from build123d import *

# Parameters (mm, degrees)
F1_DEPTH = 400
F2_R     = 15
F3_R     = 15


with BuildPart() as f1:
    # F0 (on Top) → F1 (new body)
    with BuildSketch(Plane.XY):
        Polygon((0, 400), (0, 0), (40, 0), (40, 360), (400, 360), (400, 400), align=None)
    extrude(amount=F1_DEPTH)

    # F2
    f2_edges = [f1.edges().sort_by_distance(p)[0] for p in [
        (40, 0, 200),
        (0, 0, 200),
        (400, 360, 200),
        (400, 400, 200),
    ]]
    fillet(f2_edges, radius=F2_R)

    # F3
    f3_edges = [f1.edges().sort_by_distance(p)[0] for p in [
        (0, 400, 200),
    ]]
    fillet(f3_edges, radius=F3_R)


solid = f1.part
The model under review builds one solid part; all positions refer to its coordinate system, in mm. A direction names the side the tool comes from. Give positions to 0.01 mm unless a question says otherwise; leave off trailing zeros. Write each loop counter-clockwise with the first axis right and the second up, starting at its lowest first coordinate (ties: lowest second). Pieces come first, ordered by that corner, then holes.
1. Add section C-C, the plane y = 223.5. Write out the cut boundary in (x, z), plus the area to 3 significant figures.
2. For P1, Ø3, axis at y = 188.5, z = 349.5, coming from the +X side; P2, Ø3, axis at x = 295, z = 222, coming from the -Y side, all flat-tipped, find the tip position at first contact; note any pin that passes through.
3. Tool access review of faces 1 (the flat face through (210, 360, 197)), 2 (the flat face through (36, 290, 400)): name each direction out of +Z, -Z, +X, -X, +Y, -Y from which nothing blocks a thin tool from reaching the whole face with its end or side.
4. Add section B-B, the plane x = 374. Write out the cut boundary in (y, z).
5. Add section A-A, the plane z = 108. Write out the cut boundary in (x, y).
6. Wall thickness on L1, parallel to Y at x = 368.5, z = 47.5; L2, parallel to X at y = 172, z = 380: over which ranges is each line inside the solid? List them lowest first.
Worked answers:
1. outline: (0, 0) - (40, 0) - (40, 400) - (0, 400) - close
1. area: 16,000 mm2
2. P1: stops at x = 40
2. P2: stops at y = 360
3. face 1: +Z, -Z, +X, -Y
3. face 2: +Z, +X, -X, +Y, -Y
4. outline: (360, 0) - (400, 0) - (400, 400) - (360, 400) - close
5. outline: (0, 15) arc R15 ccw to (15, 0) - (25, 0) arc R15 ccw to (40, 15) - (40, 360) - (385, 360) arc R15 ccw to (400, 375) - (400, 385) arc R15 ccw to (385, 400) - (15, 400) arc R15 ccw to (0, 385) - close
6. L1: y = 360 to 400
6. L2: x = 0 to 40
